Model file for the job. Use its own axes, mm. Give positions to 0.01 mm unless a question says otherwise; leave off trailing zeros. Write each loop counter-clockwise with the first axis right and the second up, starting at its lowest first coordinate (ties: lowest second). Pieces come first, ordered by that corner, then holes.
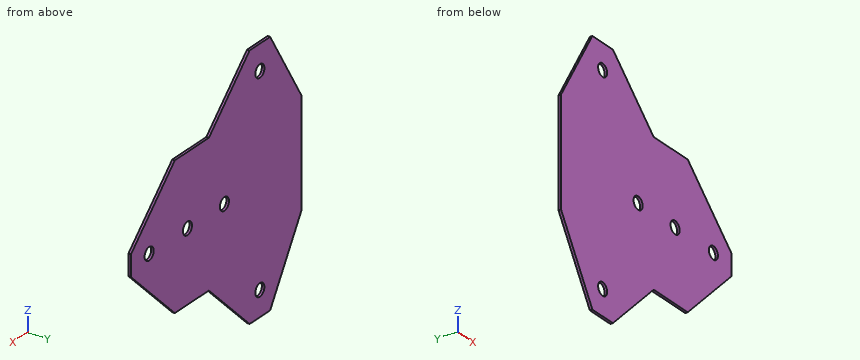
```python
from build123d import *

# Parameters (mm, degrees)
SKETCH1_R          = 2.5
BASE_FLANGE1_DEPTH = 1


# Sheet-metal steps are written as plain solids
with BuildPart() as part:
    # Sketch1 → Base-Flange1 (new body)
    with BuildSketch(Plane(origin=(0, 0, 0), x_dir=(1, 0, 0), z_dir=(0, 1, 0))):
        Polygon((5.674376272, 50), (28.180948875, 27.92), (47.02, 27.92), (71.2, 4.198289483), (71.2, -4.198289483), (47.02, -27.92), (28.180948875, -27.92), (5.674376272, -50), (-5.674376272, -50), (-23, -21), (-23, 21), (-5.674376272, 50), align=None)
        with Locations(Location((0, 40, 0), (0, 0, 270))):
            Circle(SKETCH1_R, mode=Mode.SUBTRACT)
        with Locations(Location((0, -40, 0), (0, 0, 90))):
            Circle(SKETCH1_R, mode=Mode.SUBTRACT)
        with Locations(Location((61.2, 0, 0), (0, 0, 270))):
            Circle(SKETCH1_R, mode=Mode.SUBTRACT)
        with Locations(Location((19.6, 0, 0), (0, 0, 270))):
            Circle(SKETCH1_R, mode=Mode.SUBTRACT)
        with Locations(Location((40.02, 0, 0), (0, 0, 270))):
            Circle(SKETCH1_R, mode=Mode.SUBTRACT)
    extrude(amount=-BASE_FLANGE1_DEPTH)


solid = part.part
```
1. Slice it at A-A, the plane x = 0. Write the cut outline in (y, z).
Calculated:
outline: (-1, -50) - (0, -50) - (0, -42.5) - (-1, -42.5) - close; (-1, -37.5) - (0, -37.5) - (0, 37.5) - (-1, 37.5) - close; (-1, 42.5) - (0, 42.5) - (0, 50) - (-1, 50) - close
2. Slice it at C-C, the plane x = 40.02. Write the cut outline in (y, z).
Calculated:
outline: (-1, -27.92) - (0, -27.92) - (0, -2.5) - (-1, -2.5) - close; (-1, 2.5) - (0, 2.5) - (0, 27.92) - (-1, 27.92) - close
3. Slice it at D-D, the plane z = -40. Write the cut outline in (x, y).
Calculated:
outline: (-11.65, -1) - (-2.5, -1) - (-2.5, 0) - (-11.65, 0) - close; (2.5, -1) - (15.87, -1) - (15.87, 0) - (2.5, 0) - close
4. Probe probe 1 along X at (y, z) = (-0.45, -41.5); probe 2 along Z at (x, y) = (46, -0.25); probe 3 along X at (y, z) = (-0.9, -38.5). List the from-to ranges inside material, lowest first.
Calculated:
probe 1: x = -10.75 to -2, 2 to 14.34
probe 2: z = -27.92 to 27.92
probe 3: x = -12.54 to -2, 2 to 17.4
5. Pin check, flat tip, straight feed: P1, Ø0.5, axis at x = 40, y = -0.5, coming from the +Z side. Stop position of the tip, or through.
Calculated:
P1: stops at z = 27.92
6. Slice it at B-B, the plane y = -0.5. Write the cut outline in (x, z), and give its area (3 significant figures).
Calculated:
outline: (-23, -21) - (-5.67, -50) - (5.67, -50) - (28.18, -27.92) - (47.02, -27.92) - (71.2, -4.2) - (71.2, 4.2) - (47.02, 27.92) - (28.18, 27.92) - (5.67, 50) - (-5.67, 50) - (-23, 21) - close; hole circle Ø5 at (0, -40); hole circle Ø5 at (0, 40); hole circle Ø5 at (19.6, 0); hole circle Ø5 at (40.02, 0); hole circle Ø5 at (61.2, 0)
area: 5,850 mm2
